Input: dimensioned drawing with shaded views. Units: mm. Origin: part minimum x, y, z. Round coordinates to 2 decimals unless told otherwise and drop trailing zeros. Order: outer loops, then holes, each group sorted by start corner. A loop starts at its lowest first (then second) coordinate and runs counter-clockwise, first axis right, second up.
Item 1: Cut plane A-A on y = 52.5. Output: boundary loops of the cut face in (x, z), then the cut area to 3 significant figures.
Item 2: Cut plane D-D on y = 40. Output: boundary loops of the cut face in (x, z).
Item 3: Line query: L1, parallel to Y at x = 7.5, z = 1.3; L2, parallel to Y at x = 7.5, z = 2.85 (1 decimal); L3, parallel to Y at x = 7.5, z = 3.1. Output: solid intervals per line, ascending.
Item 4: Cut plane C-C on z = 0.7. Output: boundary loops of the cut face in (x, y), then the cut area to 3 significant figures.
Item 5: Mould query, pull axis X, two halves, no side actions, for the marked faces 1, 2, 3 and 4. Classes: released by +X, released by -X, zero draft, split by the parting line, or undercut.
Item 6: Cut plane B-B on x = 7.5. Give the number of separate pieces and of enclosed holes in the cut face, then the cut area to 3 significant figures.
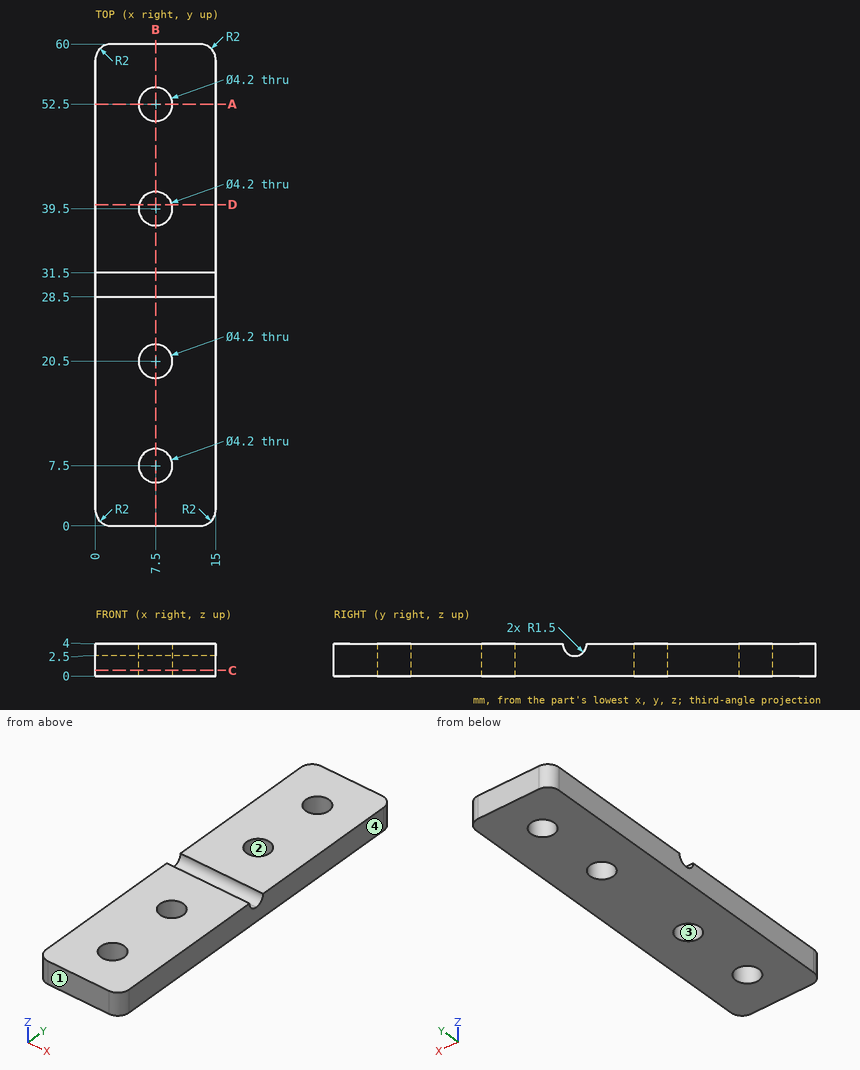
From the geometry:
1. outline: (0, 0) - (5.4, 0) - (5.4, 4) - (0, 4) - close; (9.6, 0) - (15, 0) - (15, 4) - (9.6, 4) - close
1. area: 43.2 mm2
2. outline: (0, 0) - (5.46, 0) - (5.46, 4) - (0, 4) - close; (9.54, 0) - (15, 0) - (15, 4) - (9.54, 4) - close
3. L1: y = 0 to 5.4, 9.6 to 18.4, 22.6 to 37.4, 41.6 to 50.4, 54.6 to 60
3. L2: y = 0 to 5.4, 9.6 to 18.4, 22.6 to 29, 31 to 37.4, 41.6 to 50.4, 54.6 to 60
3. L3: y = 0 to 5.4, 9.6 to 18.4, 22.6 to 28.8, 31.2 to 37.4, 41.6 to 50.4, 54.6 to 60
4. outline: (0, 2) arc R2 ccw to (2, 0) - (13, 0) arc R2 ccw to (15, 2) - (15, 58) arc R2 ccw to (13, 60) - (2, 60) arc R2 ccw to (0, 58) - close; hole circle Ø4.2 at (7.5, 7.5); hole circle Ø4.2 at (7.5, 20.5); hole circle Ø4.2 at (7.5, 39.5); hole circle Ø4.2 at (7.5, 52.5)
4. area: 841 mm2
5. face 1: zero draft
5. face 2: undercut
5. face 3: undercut
5. face 4: released by +X
6. separate pieces: 5
6. enclosed holes: 0
6. area: 169 mm2
